Build history of the part. All positions in model axes, mm. Round coordinates to 2 decimals unless told otherwise and drop trailing zeros. Write each loop counter-clockwise with the first axis right and the second up, starting at its lowest first coordinate (ties: lowest second). Pieces come first, ordered by that corner, then holes. Notation, with made-up numbers: (-17, 14.25) -> (35, 14.25) arc R11 ccw to (35, 31.25) -> close; hole circle Ø11 at (42.5, 45.5). An arc over 180 degrees is marked (long way). One line per question, with ' | ' between items.
Autodesk Inventor part; units mm, degrees
ref_plane "YZ Plane" through (0, 0, 0) normal (1, 0, 0) x (0, 1, 0)
ref_plane "XZ Plane" through (0, 0, 0) normal (0, 1, 0) x (-1, 0, 0)
ref_plane "XY Plane" through (0, 0, 0) normal (0, 0, 1) x (1, 0, 0)
sketch "Sketch1" plane through (0, 0, 0) normal (1, 0, 0) x (0, 1, 0)
  circle A0 centre (0, 0) radius 21.25
  circle A1 centre (0, 0) radius 26
  circle A2 centre (0, 21.25) radius 2
  circle A3 centre (-20.21, 6.5666) radius 2
  circle A4 centre (-12.4904, -17.1916) radius 2
  circle A5 centre (12.4904, -17.1916) radius 2
  circle A6 centre (20.21, 6.5666) radius 2
  dimension "d0" = 42.5
  dimension "d1" = 52
  dimension "d2" = 4
  dimension "d5" = 360
extrude "Extrusion1" add sketch "Sketch1" along normal blind 2 contours A0 A5 A4 A3 A2 A6 | A1
properties part number "antenna_plate"
(1) Slice it at A-A (y = 0). Write the cut outline in (x, z).
Calculated:
outline: (0, -26) -> (2, -26) -> (2, 19.25) -> (0, 19.25) -> close; (0, 23.25) -> (2, 23.25) -> (2, 26) -> (0, 26) -> close
(2) Slice it at C-C (x = 0.65). Write the cut outline in (y, z), then the cut area to 3 significant figures.
Calculated:
outline: circle Ø52 at (0, 0); hole circle Ø4 at (-20.21, 6.57); hole circle Ø4 at (-12.49, -17.19); hole circle Ø4 at (0, 21.25); hole circle Ø4 at (12.49, -17.19); hole circle Ø4 at (20.21, 6.57) | area: 2,060 mm2
(3) Wall check: line 1 (Z direction, x = 1.1, y = 0); line 2 (Z direction, x = 0.9, y = -20.21); line 3 (Y direction, x = 1.4, z = 19.5). Give the ranges that are in metal, low to high. Write a range as from..to.
Calculated:
line 1: -26..19.25, 23.25..26 | line 2: -16.36..4.57, 8.57..16.36 | line 3: -17.2..-0.97, 0.97..17.2
(4) Slice it at B-B (z = 7.5). Write the cut outline in (x, y), then the cut area to 3 significant figures.
Calculated:
outline: (0, -24.89) -> (2, -24.89) -> (2, -21.98) -> (0, -21.98) -> close; (0, -18.44) -> (2, -18.44) -> (2, 18.44) -> (0, 18.44) -> close; (0, 21.98) -> (2, 21.98) -> (2, 24.89) -> (0, 24.89) -> close | area: 85.4 mm2
(5) Slice it at D-D (z = 21.25). Write the cut outline in (x, y).
Calculated:
outline: (0, -14.98) -> (2, -14.98) -> (2, -2) -> (0, -2) -> close; (0, 2) -> (2, 2) -> (2, 14.98) -> (0, 14.98) -> close
(6) Mould opens along Z. For faces 1 (the flat face through (2, 0, 0)), 2 (the cylindrical face through (0.986, -20.633, 15.821)), 3 (the cylindrical face through (0.986, -0.26, 19.267)) say: pulls with the +Z half, pulls with the -Z half, needs draft (parallel to the pull), parting line crosses it, or undercut.
Calculated:
face 1: needs draft | face 2: parting line crosses it | face 3: undercut
